Job drawing, mm, ordinate dimensions from the low corner. One solid piece. Give positions to 0.01 mm unless a question says otherwise; leave off trailing zeros. Loops run counter-clockwise (first coordinate to the right, second up) from the corner with the lowest first, then second, coordinate; pieces in that order, holes last. Notation, with made-up numbers: (65.5, 80) -> (103.5, 80) arc R16 ccw to (103.5, 87) -> close; hole circle Ø2 at (42.25, -37). An arc over 180 degrees is marked (long way). Use one line per item in the form item = value.
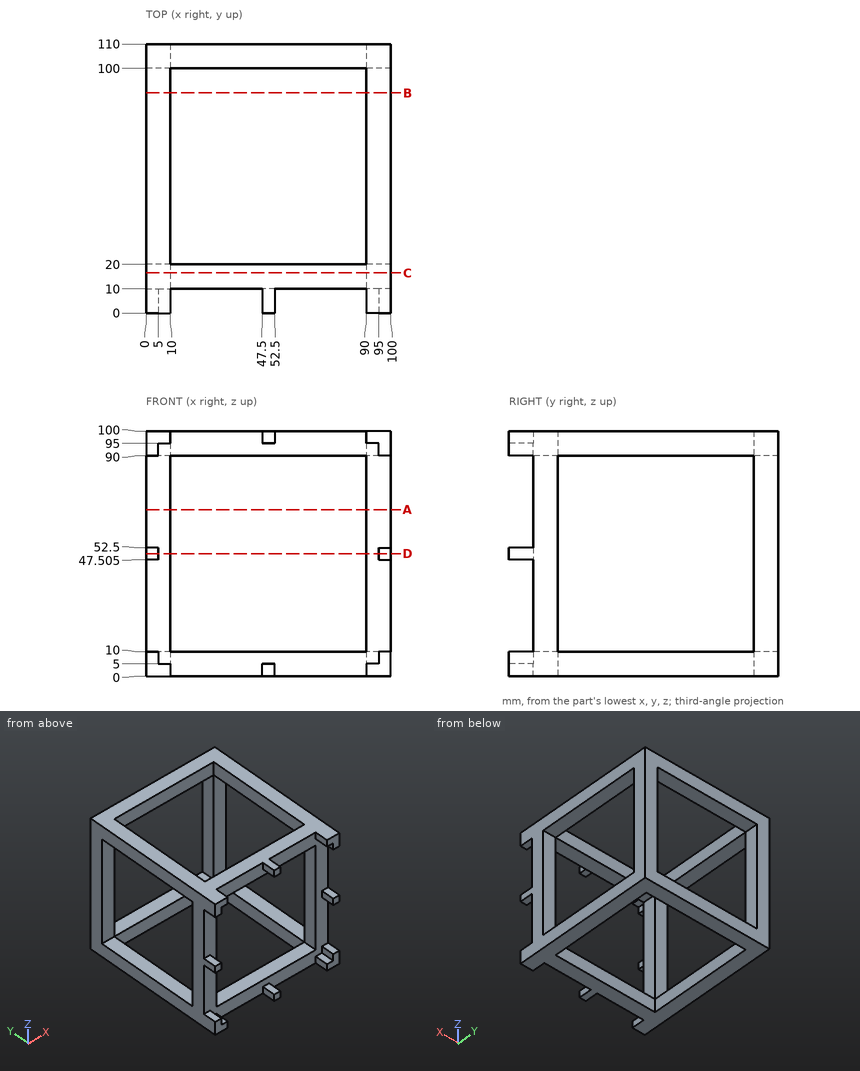
1. Cut at D-D, the plane z = 50. Write the cut outline in (x, y), then the cut area to 3 significant figures.
Result sheet:
outline = (0, 0) -> (5, 0) -> (5, 10) -> (10, 10) -> (10, 20) -> (0, 20) -> close; (0, 100) -> (10, 100) -> (10, 110) -> (0, 110) -> close; (90, 10) -> (95, 10) -> (95, 0) -> (100, 0) -> (100, 20) -> (90, 20) -> close; (90, 100) -> (100, 100) -> (100, 110) -> (90, 110) -> close
area = 500 mm^2
2. Cut at B-B, the plane y = 90. Write the cut outline in (x, z).
Result sheet:
outline = (0, 0) -> (10, 0) -> (10, 10) -> (0, 10) -> close; (0, 90) -> (10, 90) -> (10, 100) -> (0, 100) -> close; (90, 0) -> (100, 0) -> (100, 10) -> (90, 10) -> close; (90, 90) -> (100, 90) -> (100, 100) -> (90, 100) -> close
3. Cut at A-A, the plane z = 68. Write the cut outline in (x, y).
Result sheet:
outline = (0, 10) -> (10, 10) -> (10, 20) -> (0, 20) -> close; (0, 100) -> (10, 100) -> (10, 110) -> (0, 110) -> close; (90, 10) -> (100, 10) -> (100, 20) -> (90, 20) -> close; (90, 100) -> (100, 100) -> (100, 110) -> (90, 110) -> close
4. Drop a flat-ended pin along its axis: P1, Ø10, axis at x = 61, z = 14, coming from the -Y side. Give the stop position or say it passes through.
Result sheet:
P1 = 10
5. Drill centre lines: line 1 (Y direction, x = 23.5, z = 9); line 2 (X direction, y = 12.5, z = 17). Where is each one in solid material? Low to high.
Result sheet:
line_1 = 10 to 20, 100 to 110
line_2 = 0 to 10, 90 to 100
6. Cut at C-C, the plane y = 16.5. Write the cut outline in (x, z).
Result sheet:
outline = (0, 0) -> (100, 0) -> (100, 100) -> (0, 100) -> close; hole (10, 10) -> (90, 10) -> (90, 90) -> (10, 90) -> close
